Autodesk Inventor part; units mm, degrees
ref_plane "Work Plane1" through (0, 4.75, 0) normal (0, 1, 0) x (-1, 0, 0)
ref_plane "YZ Plane" through (0, 0, 0) normal (1, 0, 0) x (0, 1, 0)
ref_plane "XY Plane" through (0, 0, 0) normal (0, 0, 1) x (1, 0, 0)
sketch "Sketch1" plane through (0, 0, 0) normal (0, 0, 1) x (1, 0, 0)
  arc A0 (8.2491, -5.6527) -> (-8.2509, -5.65) centre (0, 0) ccw
  arc A1 (-6.5018, -19) -> (6.4982, -19) centre (-0.0018, -19) ccw
  circle A2 centre (0, 0) radius 4.75
  line L0 (-6.5018, -19) -> (-6.5018, -11.3)
  line L1 (6.4982, -19) -> (6.4982, -11.3053)
  arc A3 (-6.5018, -11.3) -> (-8.2509, -5.65) centre (-16.5018, -11.3) ccw
  arc A4 (8.2491, -5.6527) -> (6.4982, -11.3053) centre (16.4982, -11.3053) ccw
  point P0 (-6.5018, -7.5978)
  point P1 (6.4982, -7.6009)
  point P2 (-6.9491, -8.3427)
  dimension "d0" = 20
  dimension "d1" = 9.5
  dimension "d2" = 13
  dimension "d3" = 19
  dimension "d4" = 10
  dimension "d6" = 7.7
extrude "Extrusion1" add sketch "Sketch1" along normal blind 8
sketch "Sketch2" plane through (0, 0, 8) normal (0, 0, 1) x (1, 0, 0)
  arc A0 (-6.5018, -19) -> (6.4982, -19) centre (-0.0018, -19) ccw
hole "Hole1" at (-0.0018, -19, 8) direction (0, 0, -1) diameter 4.134 end through all
sketch "Sketch3" plane through (0, 0, 8) normal (0, 0, 1) x (1, 0, 0)
  circle A0 centre (0, 0) radius 4.75
  circle A1 centre (0, 0) radius 4.75
extrude "Extrusion2" add sketch "Sketch3" against normal blind 95
chamfer "Chamfer1" distance 0.5 angle 45 13 edges at (0.0016, 10, 8) (-6.9491, -8.3427, 8) (-6.5018, -15.15, 8) (-0.0018, -25.5, 8) (6.4982, -15.1527, 8) (6.9459, -8.3465, 8) (-4.75, 0, -87) (-0.0018, -25.5, 0) (6.4982, -15.1527, 0) (6.9459, -8.3465, 0) (0.0016, 10, 0) (-6.9491, -8.3427, 0) (-6.5018, -15.15, 0)
ref_plane "Work Plane1" through (0, 4.75, 0) normal (0, 1, 0) x (-1, 0, 0)
sketch "Sketch4" plane through (0, 4.75, 0) normal (0, 1, 0) x (-1, 0, 0)
  circle A0 centre (0, -63.5) radius 1.5
  line L0 (-4.75, -87) -> (4.75, -87)
  point P0 (0, 0)
  point P1 (0, -87)
  dimension "d22" = 3
  dimension "d23" = 23.5
extrude "Extrusion3" cut sketch "Sketch4" against normal through all
properties part number "Crankshaft" material "Steel AISI 1020 107 HR"
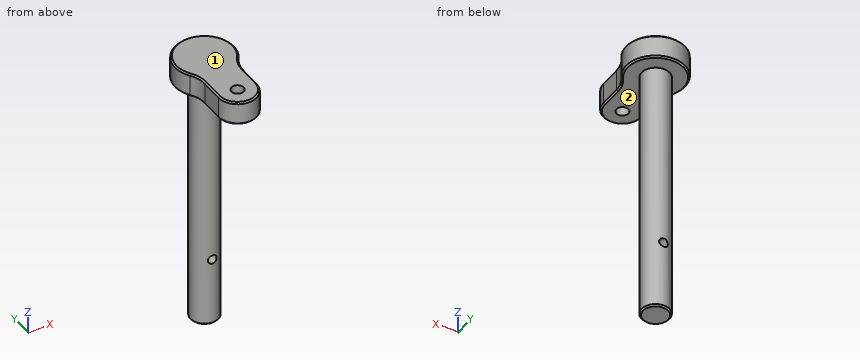
CAD build for the part. Positions are in the model's coordinates, mm. Face numbers are marked on the shaded views. A direction names the side the tool comes from. Round coordinates to 2 decimals unless told otherwise and drop trailing zeros. Order: outer loops, then holes, each group sorted by start corner. A loop starts at its lowest first (then second) coordinate and runs counter-clockwise, first axis right, second up. Notation, with made-up numbers: (60, 40) - (110, 40) arc R27 cw to (110, 73) - close; hole circle Ø6 at (43, -3). An arc over 180 degrees is marked (long way). Answer as CSV lines item,"result". Start each with the question number.
1. Drill centre lines: L1, parallel to X at y = -19, z = 5; L2, parallel to Z at x = 5, y = -1.5; L3, parallel to Z at x = 0, y = -1.5. Where is each one in solid material? Low to high. Write a range as [from, to].
2. Pin check, flat tips, straight feed: pin 1 (12 mm diameter, centred on x = 1, z = -60, fed in from +Y); pin 2 (2 mm diameter, centred on y = -15, z = 5, fed in from -X); pin 3 (10 mm diameter, centred on x = -3, z = -63.5, fed in from -Y); pin 4 (1.8 mm diameter, centred on x = 0, z = -63.5, fed in from +Y). Stop position of each tip, or through.
3. Tool access for the marked faces 1 and 2: list every direction of +Z, -Z, +X, -X, +Y, -Y with a clear straight run to the whole face (end or side of a thin tool).
4. Saw through at A-A, the plane z = -63.5. Write the cut outline in (x, y).
5. Saw through at B-B, the plane z = -39. Write the cut outline in (x, y), and give its area (3 significant figures).
Model answer:
1,L1,"x = [-6.5, -2.07], [2.07, 6.5]"
1,L2,"z = [0, 8]"
1,L3,"z = [-87, -65], [-62, 8]"
2,pin 1,"stops at y = 4.75"
2,pin 2,"stops at x = -6.5"
2,pin 3,"stops at y = -4.75"
2,pin 4,"passes through"
3,face 1,"+Z, +X, -X, +Y, -Y"
3,face 2,"-Z"
4,outline,"(-1.5, -4.51) - (-1.5, 4.51) arc R4.75 ccw to start; (1.5, -4.51) arc R4.75 ccw to (1.5, 4.51) - close"
5,outline,"circle Ø9.5 at (0, 0)"
5,area,"70.9 mm²"
